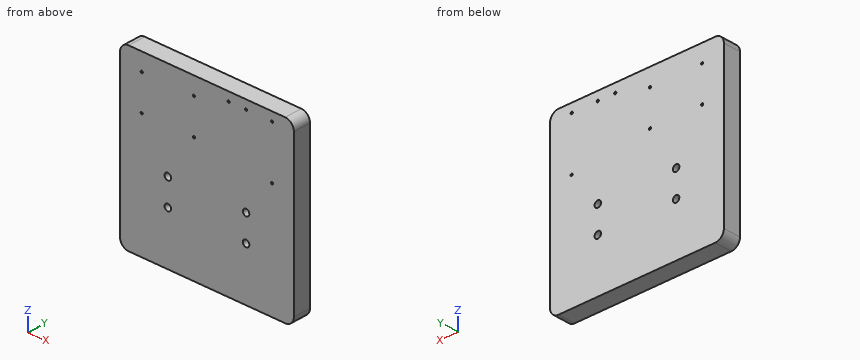
from build123d import *

# Parameters (mm, degrees)
CROQUIS1_W              = 200
CROQUIS1_H              = 200
SALIENTE_EXTRUIR1_DEPTH = 20
REDONDEO1_R             = 10
CROQUIS5_W              = 120
CROQUIS5_H              = 80
SALIENTE_EXTRUIR3_DEPTH = 20
CROQUIS3_R              = 3.75
CORTAR_EXTRUIR2_DEPTH   = 21
CROQUIS6_R              = 1.25
CORTAR_EXTRUIR3_DEPTH   = 21


with BuildPart() as part:
    # Croquis1 → Saliente-Extruir1 (new body)
    with BuildSketch(Plane(origin=(0, 0, 0), x_dir=(1, 0, 0), z_dir=(0, 1, 0))):
        Rectangle(CROQUIS1_W, CROQUIS1_H)
    extrude(amount=SALIENTE_EXTRUIR1_DEPTH)

    # Redondeo1
    redondeo1_edges = [part.edges().sort_by_distance(p)[0] for p in [
        (100, 10, 100),
        (-100, 10, 100),
        (-100, 10, -100),
        (100, 10, -100),
    ]]
    fillet(redondeo1_edges, radius=REDONDEO1_R)

    # Croquis5 → Saliente-Extruir3 (add)
    with BuildSketch(Plane(origin=(0, 20, 0), x_dir=(1, 0, 0), z_dir=(0, 1, 0))):
        with Locations((0, 20)):
            Rectangle(CROQUIS5_W, CROQUIS5_H)
    extrude(amount=-SALIENTE_EXTRUIR3_DEPTH)

    # Croquis3 → Cortar-Extruir2 (cut, through all)
    with BuildSketch(Plane(origin=(0, 20, 0), x_dir=(1, 0, 0), z_dir=(0, 1, 0))):
        with Locations((-45, 10)):
            Circle(CROQUIS3_R)
        with Locations((45, 10)):
            Circle(CROQUIS3_R)
    cortar_extruir2 = extrude(amount=-CORTAR_EXTRUIR2_DEPTH, mode=Mode.SUBTRACT)

    # Simetría3: Cortar-Extruir2 across plane
    add(cortar_extruir2.mirror(Plane.XY.offset(-25)), mode=Mode.SUBTRACT)

    # Croquis6 → Cortar-Extruir3 (cut, through all)
    with BuildSketch(Plane(origin=(0, 20, 0), x_dir=(1, 0, 0), z_dir=(0, 1, 0))):
        with Locations((75, -90)):
            Circle(CROQUIS6_R)
        with Locations((75, -30)):
            Circle(CROQUIS6_R)
        with Locations((45, -90)):
            Circle(CROQUIS6_R)
        with Locations((25, -90)):
            Circle(CROQUIS6_R)
        with Locations((-15, -80)):
            Circle(CROQUIS6_R)
        with Locations((-15, -40)):
            Circle(CROQUIS6_R)
        with Locations((-75, -40)):
            Circle(CROQUIS6_R)
        with Locations((-75, -80)):
            Circle(CROQUIS6_R)
    extrude(amount=-CORTAR_EXTRUIR3_DEPTH, mode=Mode.SUBTRACT)


solid = part.part
Could you check a few things on this model? Use its own coordinates, in mm. Give positions to 0.01 mm unless a question says otherwise; leave off trailing zeros. Order: outer loops, then holes, each group sorted by start corner. A loop starts at its lowest first (then second) coordinate and runs counter-clockwise, first axis right, second up. Notation, with made-up numbers: (65, 85.5) - (105, 85.5) arc R36 ccw to (105, 124.5) - close; hole circle Ø7 at (66.5, 72). An arc over 180 degrees is marked (long way). Return JSON: item names as keys, results as strings. Group by question number.
Q1. Suppose I cut it at A-A, the plane z = -10. Please give me the cut outline in (x, y), and give its area (3 significant figures).
Q2. Please list where these lines run through material, in increasing order: line 1 along Z through (x, y) = (45, 7.75); line 2 along Z through (x, y) = (-15, 5.75); line 3 along X through (y, z) = (13.25, -10). Write a range as [from, to].
Q3. Will this pin go through, and if not, where does the flat tip stop? pin 1 Ø2 at (x, z) = (-75, 80) entering from +Y.
Resolved:
{
 "1": {"outline": "(-100, 0) - (-48.75, 0) - (-48.75, 20) - (-100, 20) - close; (-41.25, 0) - (41.25, 0) - (41.25, 20) - (-41.25, 20) - close; (48.75, 0) - (100, 0) - (100, 20) - (48.75, 20) - close", "area": "3,700 mm2"},
 "2": {"line 1": "z = [-100, -43.75], [-36.25, -13.75], [-6.25, 88.75], [91.25, 100]", "line 2": "z = [-100, 38.75], [41.25, 78.75], [81.25, 100]", "line 3": "x = [-100, -48.75], [-41.25, 41.25], [48.75, 100]"},
 "3": {"pin 1": "passes through"}
}
